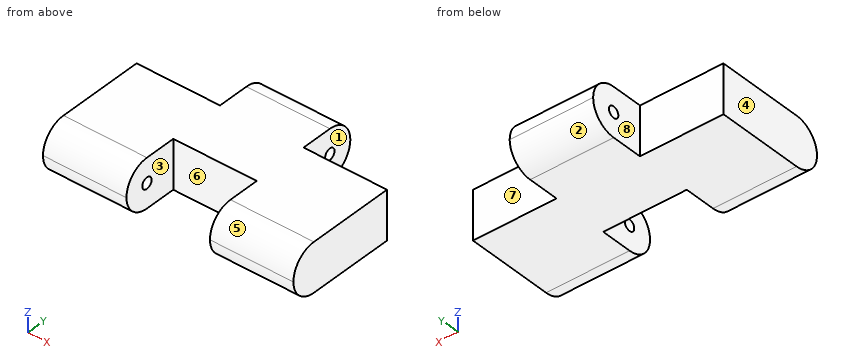
```python
from build123d import *

# Parameters (mm, degrees)
F1_DEPTH = 22.225
F2_R     = 22.22499
F3_R     = 5.08
F4_DEPTH = 114.301
F5_DEPTH = 114.301
F6_R     = 5.08
F7_DEPTH = 63.5


# Not quite as in the source:
# - a fillet or chamfer is up to 0.001 mm smaller than in the source, because OpenCascade refuses the exact size


with BuildPart() as f1:
    # F0 (on Top) → F1 (new body, symmetric)
    with BuildSketch(Plane.XY):
        Polygon((38.1, 40.6722736142), (0, 40.6722736142), (-38.1, 40.6722736142), (-38.1, -10.1277263858), (-114.3, -10.1277263858), (-114.3, -111.7277263858), (-38.1, -111.7277263858), (-38.1, -60.9277263858), (38.1, -60.9277263858), (38.1, -111.7277263858), (114.3, -111.7277263858), (114.3, -10.1277263858), (38.1, -10.1277263858), align=None)
    extrude(amount=F1_DEPTH, both=True)

    # F2 (radius 22.225 in the source; OpenCascade refuses exactly that, so slightly less here)
    f2_edges = [f1.edges().sort_by_distance(p)[0] for p in [
        (-76.2, -111.727726, 22.225),
        (-76.2, -111.727726, -22.225),
        (76.2, -111.727726, 22.225),
        (76.2, -111.727726, -22.225),
        (0, 40.672274, 22.225),
        (0, 40.672274, -22.225),
    ]]
    fillet(f2_edges, radius=F2_R)

    # F3 (on Right) → F4 (cut, through all)
    with BuildSketch(Plane.YZ):
        with Locations((18.4472736142, 0)):
            Circle(F3_R)
    extrude(amount=-F4_DEPTH, mode=Mode.SUBTRACT)

    # F3 (on Right) → F5 (cut, through all)
    with BuildSketch(Plane.YZ):
        with Locations((18.4472736142, 0)):
            Circle(F3_R)
    extrude(amount=F5_DEPTH, mode=Mode.SUBTRACT)

    # F6 (on Right) → F7 (cut, symmetric)
    with BuildSketch(Plane.YZ):
        with Locations((-89.5027263858, 0)):
            Circle(F6_R)
    extrude(amount=F7_DEPTH, both=True, mode=Mode.SUBTRACT)


solid = f1.part
```
Can you work these out from the model? Positions are in its coordinate system, mm. Face numbers are marked on the shaded views. A direction names the side the tool comes from. Round coordinates to 2 decimals unless told otherwise and drop trailing zeros. Loops run counter-clockwise (first coordinate to the right, second up) from the corner with the lowest first, then second, coordinate; pieces in that order, holes last. Notation, with made-up numbers: M -27.75,19 L 14.25,19 A23 ccw 14.25,32 Z; hole C 58,56 d7. An arc over 180 degrees is marked long. Answer in a Markdown table with one row per item.
1. If we section it at D-D, the plane y = 10: Please give me the cut outline in (x, z) (3 decimals), plus the area to 3 significant figures.
Established:
| item | result |
|---|---|
| outline | M -38.1,-22.225 L 38.1,-22.225 L 38.1,22.225 L -38.1,22.225 Z |
| area | 3,390 mm² |
2. I'm going to push flat-ended pins straight in: pin 1 Ø3 at (y, z) = (15, 12.5) entering from +X; pin 2 Ø22 at (x, z) = (86, -5) entering from +Y; pin 3 Ø11.5 at (y, z) = (18.45, 0) entering from -X. Where does each tip first touch, or does it pass through?
Established:
| item | result |
|---|---|
| pin 1 | x = 38.1 |
| pin 2 | y = -10.13 |
| pin 3 | x = -38.1 |
3. Please list where these lines run through material, in increasing order: line 1 (X direction, y = -72, z = -13); line 2 (Y direction, x = 3.5, z = 0); line 3 (Y direction, x = 99.5, z = -1.5). Write a range as from..to.
Established:
| item | result |
|---|---|
| line 1 | -114.3..-38.1, 38.1..114.3 |
| line 2 | -60.93..13.37, 23.53..40.67 |
| line 3 | -111.68..-10.13 |
4. Thinking about a two-plate mould opening in X: for the marked faces 1, 2 and 3, which applies, pulls with the +X half, pulls with the -X half, needs draft (parallel to the pull), parting line crosses it, or undercut?
Established:
| item | result |
|---|---|
| face 1 | pulls with the +X half |
| face 2 | needs draft |
| face 3 | undercut |
5. If we section it at B-B, the plane y = -99: Please give me the cut outline in (x, z), plus the area to 3 significant figures.
Established:
| item | result |
|---|---|
| outline | M -114.3,-20.09 L -38.1,-20.09 L -38.1,20.09 L -114.3,20.09 Z; M 38.1,-20.09 L 114.3,-20.09 L 114.3,20.09 L 38.1,20.09 Z |
| area | 6,120 mm² |
6. On a 3-axis mill with a long thin cutter (end or side, diameter ignored), from which of +Z, -Z, +X, -X, +Y, -Y can I reach the whole of each face in a straight line? I mean the marked faces 4, 5, 6, 7 and 8. Say none if no direction works.
Established:
| item | result |
|---|---|
| face 4 | +Z, -Z, -X, +Y, -Y |
| face 5 | +Z, +X, -X, -Y |
| face 6 | +Z, -Z, -Y |
| face 7 | +Z, -Z, +X, +Y |
| face 8 | +Z, -Z, -X, +Y |
